```python
from build123d import *

# Parameters (mm, degrees)
SKETCH1_W                   = 79.5
SKETCH1_H                   = 79.5
SKETCH1_W_2                 = 54.5
SKETCH1_H_2                 = 54.5
BOSS_EXTRUDE1_DEPTH         = 12.7
CHAMFER2_SIZE               = 4
SKETCH2_W                   = 34.5
SKETCH2_H                   = 5
SKETCH2_H_2                 = 0.75
CUT_EXTRUDE1_DEPTH          = 64.41462765
BOSS_EXTRUDE2_DEPTH         = 12.7
CUT_EXTRUDE2_DEPTH          = 3
CUT_EXTRUDE3_DEPTH          = 121.131604917
CHAMFER5_SIZE               = 0.5
CHAMFER5_SIZE2              = 0.866025404
TAP_DRILL_FOR_M5X0_8_TAP3_D = 4.2
CUT_EXTRUDE4_DEPTH          = 74.291984555
FILLET1_R                   = 1.5
FILLET2_R                   = 1.5
FILLET3_R                   = 1.5
CHAMFER4_SIZE               = 1


with BuildPart() as part:
    # Sketch1 → Boss-Extrude1 (new body)
    with BuildSketch(Plane.XY):
        with Locations((0, 8)):
            Rectangle(SKETCH1_W, SKETCH1_H)
        Rectangle(SKETCH1_W_2, SKETCH1_H_2, mode=Mode.SUBTRACT)
    extrude(amount=BOSS_EXTRUDE1_DEPTH)

    # Chamfer2
    chamfer2_edges = [part.edges().sort_by_distance(p)[0] for p in [
        (39.75, -31.75, 6.35),
        (-39.75, -31.75, 6.35),
        (-39.75, 47.75, 6.35),
        (39.75, 47.75, 6.35),
    ]]
    chamfer(chamfer2_edges, length=CHAMFER2_SIZE)

    # Sketch2 → Cut-Extrude1 (cut, through all)
    with BuildSketch(Plane.XY.offset(12.7)):
        with BuildLine():
            Line((-27.25, 27.25), (-25.5, 27.25))
            Line((-25.5, 27.25), (-25.5, 43.25))
            Line((-25.5, 43.25), (-29.25, 43.25))
            ThreePointArc((-29.25, 43.25), (-33.492640687, 41.492640687), (-35.25, 37.25))
            Line((-35.25, 37.25), (-35.25, 0.75))
            Line((-35.25, 0.75), (-27.25, 0.75))
            Line((-27.25, 0.75), (-27.25, 27.25))
        make_face()
        with Locations((0, 29.75)):
            Rectangle(SKETCH2_W, SKETCH2_H)
        with BuildLine():
            Line((25.5, 43.25), (25.5, 27.25))
            Line((25.5, 27.25), (27.25, 27.25))
            Line((27.25, 27.25), (27.25, 0.75))
            Line((27.25, 0.75), (35.25, 0.75))
            Line((35.25, 0.75), (35.25, 37.25))
            ThreePointArc((35.25, 37.25), (33.492640687, 41.492640687), (29.25, 43.25))
            Line((29.25, 43.25), (25.5, 43.25))
        make_face()
        with Locations((0, -27.625)):
            Rectangle(SKETCH2_W, SKETCH2_H_2)
    extrude(amount=-CUT_EXTRUDE1_DEPTH, mode=Mode.SUBTRACT)

    # Sketch5 → Boss-Extrude2 (add)
    with BuildSketch(Plane.XY.offset(12.7)):
        with BuildLine():
            Line((-47.25, -31.75), (-35.75, -31.75))
            Line((-35.75, -31.75), (-39.75, -27.75))
            Line((-39.75, -27.75), (-39.75, 43.75))
            Line((-39.75, 43.75), (-35.75, 47.75))
            Line((-35.75, 47.75), (-47.25, 47.75))
            ThreePointArc((-47.25, 47.75), (-52.553300859, 45.553300859), (-54.75, 40.25))
            Line((-54.75, 40.25), (-54.75, -24.25))
            ThreePointArc((-54.75, -24.25), (-52.553300859, -29.553300859), (-47.25, -31.75))
        make_face()
        with BuildLine():
            Line((35.75, -31.75), (47.25, -31.75))
            ThreePointArc((47.25, -31.75), (52.553300859, -29.553300859), (54.75, -24.25))
            Line((54.75, -24.25), (54.75, 40.25))
            ThreePointArc((54.75, 40.25), (52.553300859, 45.553300859), (47.25, 47.75))
            Line((47.25, 47.75), (35.75, 47.75))
            Line((35.75, 47.75), (39.75, 43.75))
            Line((39.75, 43.75), (39.75, -27.75))
            Line((39.75, -27.75), (35.75, -31.75))
        make_face()
    extrude(amount=-BOSS_EXTRUDE2_DEPTH)

    # Sketch7 → Cut-Extrude2 (cut)
    with BuildSketch(Plane.XY.offset(12.7)):
        with BuildLine():
            ThreePointArc((54.75, 40.25), (52.553300859, 45.553300859), (47.25, 47.75))
            Line((47.25, 47.75), (-47.25, 47.75))
            ThreePointArc((-47.25, 47.75), (-52.553300859, 45.553300859), (-54.75, 40.25))
            Line((-54.75, 40.25), (-54.75, -24.25))
            ThreePointArc((-54.75, -24.25), (-52.553300859, -29.553300859), (-47.25, -31.75))
            Line((-47.25, -31.75), (47.25, -31.75))
            ThreePointArc((47.25, -31.75), (52.553300859, -29.553300859), (54.75, -24.25))
            Line((54.75, -24.25), (54.75, 40.25))
        make_face()
        with BuildLine():
            ThreePointArc((35.25, -21.25), (33.492640687, -25.492640687), (29.25, -27.25))
            Line((29.25, -27.25), (27.25, -27.25))
            Line((27.25, -27.25), (17.25, -27.25))
            Line((17.25, -27.25), (17.25, -28))
            Line((17.25, -28), (-17.25, -28))
            Line((-17.25, -28), (-17.25, -27.25))
            Line((-17.25, -27.25), (-27.25, -27.25))
            Line((-27.25, -27.25), (-29.25, -27.25))
            ThreePointArc((-29.25, -27.25), (-33.492640687, -25.492640687), (-35.25, -21.25))
            Line((-35.25, -21.25), (-35.25, 0.75))
            Line((-35.25, 0.75), (-35.25, 37.25))
            ThreePointArc((-35.25, 37.25), (-33.492640687, 41.492640687), (-29.25, 43.25))
            Line((-29.25, 43.25), (-25.5, 43.25))
            Line((-25.5, 43.25), (25.5, 43.25))
            Line((25.5, 43.25), (29.25, 43.25))
            ThreePointArc((29.25, 43.25), (33.492640687, 41.492640687), (35.25, 37.25))
            Line((35.25, 37.25), (35.25, 0.75))
            Line((35.25, 0.75), (35.25, -21.25))
        make_face(mode=Mode.SUBTRACT)
    extrude(amount=-CUT_EXTRUDE2_DEPTH, mode=Mode.SUBTRACT)

    # Sketch8 → Cut-Extrude3 (cut, through all)
    with BuildSketch(Plane.ZY.offset(54.75)):
        Polygon((5.628932188, -31.75), (12.7, -24.678932188), (12.7, -31.75), align=None)
        Polygon((12.7, 47.75), (5.628932188, 47.75), (12.7, 40.678932188), align=None)
    extrude(amount=-CUT_EXTRUDE3_DEPTH, mode=Mode.SUBTRACT)

    # Chamfer5
    chamfer5_edges = [part.edges().sort_by_distance(p)[0] for p in [
        (-35.25, -10.25, 12.7),
        (-34.974594209, -23.046947729, 12.7),
    ]]
    chamfer5_side = [part.faces().sort_by_distance(p)[0] for p in [
        (-31.22846957, -11.895050932, 12.7),
    ]]
    chamfer(chamfer5_edges, length=CHAMFER5_SIZE, length2=CHAMFER5_SIZE2, reference=chamfer5_side[0])

    # Tap Drill for M5x0.8 Tap3 (through all)
    with Locations(Plane.XY.offset(9.7)):
        with Locations((-45.5, 37), (-45.5, -21), (45.5, -21), (45.5, 37)):
            Hole(TAP_DRILL_FOR_M5X0_8_TAP3_D / 2)

    # Sketch11 → Cut-Extrude4 (cut, through all)
    with BuildSketch(Plane.XY.offset(9.7)):
        with BuildLine():
            Line((-38.5, 23), (-38.5, -7))
            ThreePointArc((-38.5, -7), (-44, -12.5), (-49.5, -7))
            Line((-49.5, -7), (-49.5, 23))
            ThreePointArc((-49.5, 23), (-44, 28.5), (-38.5, 23))
        make_face()
        with BuildLine():
            Line((38.5, 23), (38.5, -7))
            ThreePointArc((38.5, -7), (44, -12.5), (49.5, -7))
            Line((49.5, -7), (49.5, 23))
            ThreePointArc((49.5, 23), (44, 28.5), (38.5, 23))
        make_face()
    extrude(amount=-CUT_EXTRUDE4_DEPTH, mode=Mode.SUBTRACT)

    # Fillet1
    fillet1_edges = [part.edges().sort_by_distance(p)[0] for p in [
        (-27.25, -27.25, 4.85),
        (27.25, -27.25, 4.85),
        (-25.5, 43.25, 4.85),
        (-27.25, 0.75, 6.35),
        (-35.25, 0.75, 4.85),
        (35.25, 0.75, 4.85),
        (27.25, 0.75, 6.35),
        (25.5, 43.25, 4.85),
    ]]
    fillet(fillet1_edges, radius=FILLET1_R)

    # Fillet2
    # the kernel refuses this fillet: 1.5 mm, written as the material it adds along each edge
    with BuildSketch(Plane(origin=(17.25, -28, 12.626527452), x_dir=(0, 1, 0), z_dir=(0, 0, -1))) as fillet2_piece_1_section:
        with BuildLine():
            CenterArc((1.5, -1.299038106), FILLET2_R, 120, 60)
            Line((0, -1.299038106), (-0.03, -1.299038106))
            Line((-0.03, -1.299038106), (-0.03, 0))
            Line((-0.03, 0), (0, 0.03))
            ThreePointArc((0, 0.03), (0.375, 0.03), (0.735, 0.025980762))
            Line((0.735, 0.025980762), (0.75, 0))
        make_face()
    fillet2_piece_1 = extrude(amount=12.626527452, mode=Mode.PRIVATE)
    fillet2_piece_1 = split(fillet2_piece_1, bisect_by=Plane(origin=(16.927844244, -27.803524046, 9.7), z_dir=(0, 0, -1)), keep=Keep.TOP, mode=Mode.PRIVATE)
    fillet2_piece_1 = split(fillet2_piece_1, bisect_by=Plane(origin=(16.927844244, -30.206033858, 7.17289833), z_dir=(0, 0.7071067811865475, -0.7071067811865477)), keep=Keep.TOP, mode=Mode.PRIVATE)
    add(fillet2_piece_1)
    with BuildSketch(Plane(origin=(-17.25, -28, 12.626527452), x_dir=(1, 0, 0), z_dir=(0, 0, -1))) as fillet2_piece_2_section:
        with BuildLine():
            CenterArc((1.299038106, -1.5), FILLET2_R, 90, 60)
            Line((0, -0.75), (-0.025980762, -0.735))
            ThreePointArc((-0.025980762, -0.735), (-0.03, -0.375), (-0.03, 0))
            Line((-0.03, 0), (0, 0.03))
            Line((0, 0.03), (1.299038106, 0.03))
            Line((1.299038106, 0.03), (1.299038106, 0))
        make_face()
    fillet2_piece_2 = extrude(amount=12.626527452, mode=Mode.PRIVATE)
    fillet2_piece_2 = split(fillet2_piece_2, bisect_by=Plane(origin=(-16.927844244, -27.803524046, 9.7), z_dir=(0, 0, -1)), keep=Keep.TOP, mode=Mode.PRIVATE)
    fillet2_piece_2 = split(fillet2_piece_2, bisect_by=Plane(origin=(-16.927844244, -30.206033859, 7.172898329), z_dir=(0, 0.7071067811865475, -0.7071067811865477)), keep=Keep.TOP, mode=Mode.PRIVATE)
    add(fillet2_piece_2)

    # Fillet3
    fillet3_edges = [part.edges().sort_by_distance(p)[0] for p in [
        (-17.25, -27.25, 4.85),
        (17.25, -27.25, 4.85),
    ]]
    fillet(fillet3_edges, radius=FILLET3_R)

    # Chamfer4
    # the kernel refuses this chamfer: 1 mm, written as the material it takes off along each edge
    with BuildSketch(Plane(origin=(-27.25, -27.250615176, 12.7), x_dir=(0.027495876610585647, 0, -0.9996219169112968), z_dir=(0, 1, 0)), Plane(origin=(27.25, 1.821682988, 12.7), x_dir=(-0.027495876610585647, 0, -0.9996219169112968), z_dir=(0, -1, 0))) as chamfer4_piece_1:
        Polygon((CHAMFER4_SIZE * 0.999621916911, CHAMFER4_SIZE * 0.0274958766106), (-CHAMFER4_SIZE * 0.0274958766106, CHAMFER4_SIZE * 0.999621916911), (0, 0), align=None)
    extrude(amount=29.072298164, mode=Mode.SUBTRACT)
    with BuildSketch(Plane(origin=(-28.071682988, 27.25, 12.7), x_dir=(0, -0.027495876610585647, -0.9996219169112968), z_dir=(1, 0, 0))) as chamfer4_piece_2:
        Polygon((CHAMFER4_SIZE * 0.999621916911, CHAMFER4_SIZE * 0.0274958766106), (-CHAMFER4_SIZE * 0.0274958766106, CHAMFER4_SIZE * 0.999621916911), (0, 0), align=None)
    extrude(amount=13.393365976, mode=Mode.SUBTRACT)
    with BuildSketch(Plane(origin=(14.678317012, 27.25, 12.7), x_dir=(0, 0.9996219169112968, 0.027495876610585647), z_dir=(1, 0, 0))) as chamfer4_piece_3:
        Polygon((CHAMFER4_SIZE * 0.999621916911, -CHAMFER4_SIZE * 0.0274958766106), (-CHAMFER4_SIZE * 0.0274958766106, -CHAMFER4_SIZE * 0.999621916911), (0, 0), align=None)
    extrude(amount=13.393365976, mode=Mode.SUBTRACT)


solid = part.part
```
Geometry check sheet. Reference: the model listing, model coordinates, mm. A direction names the side the tool comes from. Coordinates: 2 decimals unless noted, no trailing zeros. Order: outer loops, then holes, each group sorted by start corner. A loop starts at its lowest first (then second) coordinate and runs counter-clockwise, first axis right, second up. Notation, with made-up numbers: (39.5, 79) - (72.5, 79) arc R17 ccw to (72.5, 93) - close; hole circle Ø3 at (1.25, 61.5). An arc over 180 degrees is marked (long way). Answer as a JSON object with one key per item and string values. Group by question number.
Item 1: Sectioned sample at A-A, the plane x = 20.5. Record the cut outline in (y, z), and give its area (3 significant figures).
Item 2: Sectioned sample at D-D, the plane z = 3. Give the number of separate pieces and of enclosed holes in the cut face, and give its area (3 significant figures).
Item 3: Sectioned sample at C-C, the plane x = 45.5. Record the cut outline in (y, z).
Item 4: Tool access check on faces 4 (the face through (32, -12, 12.7)), 5 (the face through (-38.5, 8, 5)). Record the directions out of +Z, -Z, +X, -X, +Y, -Y that give a thin tool (end or side, any length) a straight path to the whole face; none if there is none.
Item 5: Depth check by flat-ended pin: pin 1 Ø5.5 at (x, y) = (-45.5, -21) entering from -Z; pin 2 Ø0.5 at (x, z) = (-28.5, 10) entering from -Y; pin 3 Ø3.5 at (y, z) = (-14.5, 12) entering from +X; pin 4 Ø1 at (x, y) = (35.5, 5) entering from +Z. Enter the tip coordinate at first touch or a pass-through.
Item 6: Draft check along X on faces 1 (the face through (37, 11, 9.7)), 2 (the face through (0, -28, 5)), 3 (the face through (-53.346, 44.619, 3.84)). Enter one of: +X half, -X half, draft (parallel to the pull), parting line (faces both ways), or undercut.
Item 7: Sectioned sample at B-B, the plane y = 18.5. Record the cut outline in (x, z), and give its area (3 significant figures).
Item 8: Scan lines: probe 1 along Y at (x, z) = (-45.5, 7.5); probe 2 along Y at (x, z) = (23.5, 1.75); probe 3 along Y at (x, z) = (-45.5, 2). Record each from-to range of solid material in increasing order.
Resolved:
{
 "1": {"outline": "(-31.75, 0) - (-27.25, 0) - (-27.25, 9.7) - (-27.68, 9.7) - (-31.75, 5.63) - close; (27.25, 0) - (47.75, 0) - (47.75, 5.63) - (43.68, 9.7) - (43.25, 9.7) - (43.25, 10.13) - (40.68, 12.7) - (28.25, 12.7) - (27.25, 11.7) - close", "area": "270 mm^2"},
 "2": {"separate pieces": "1", "enclosed holes": "7", "area": "3,860 mm^2"},
 "3": {"outline": "(-31.75, 0) - (-23.1, 0) - (-23.1, 9.7) - (-27.68, 9.7) - (-31.75, 5.63) - close; (-18.9, 0) - (-12.29, 0) - (-12.29, 9.7) - (-18.9, 9.7) - close; (28.29, 0) - (34.9, 0) - (34.9, 9.7) - (28.29, 9.7) - close; (39.1, 0) - (47.75, 0) - (47.75, 5.63) - (43.68, 9.7) - (39.1, 9.7) - close"},
 "4": {"face 4": "+Z, +X, -X, +Y, -Y", "face 5": "+Z, -Z"},
 "5": {"pin 1": "z = 0", "pin 2": "y = -27.25", "pin 3": "x = 35.25", "pin 4": "z = 9.7"},
 "6": {"face 1": "draft", "face 2": "undercut", "face 3": "-X half"},
 "7": {"outline": "(-54.75, 0) - (-49.5, 0) - (-49.5, 9.7) - (-54.75, 9.7) - close; (-38.5, 0) - (-35.25, 0) - (-35.25, 9.7) - (-38.5, 9.7) - close; (35.25, 0) - (38.5, 0) - (38.5, 9.7) - (35.25, 9.7) - close; (49.5, 0) - (54.75, 0) - (54.75, 9.7) - (49.5, 9.7) - close", "area": "165 mm^2"},
 "8": {"probe 1": "-29.88 to -23.1, -18.9 to -12.29, 28.29 to 34.9, 39.1 to 45.88", "probe 2": "-31.75 to -27.25, 27.25 to 47.75", "probe 3": "-31.75 to -23.1, -18.9 to -12.29, 28.29 to 34.9, 39.1 to 47.75"}
}
